Study the drawing (mm; zero at the part's minimum x, y, z) and answer. Give positions to 0.01 mm unless a question says otherwise; leave off trailing zeros. Order: outer loops, then holes, each group sorted by start corner. A loop starts at its lowest first (then second) coordinate and runs counter-clockwise, first axis right, second up.
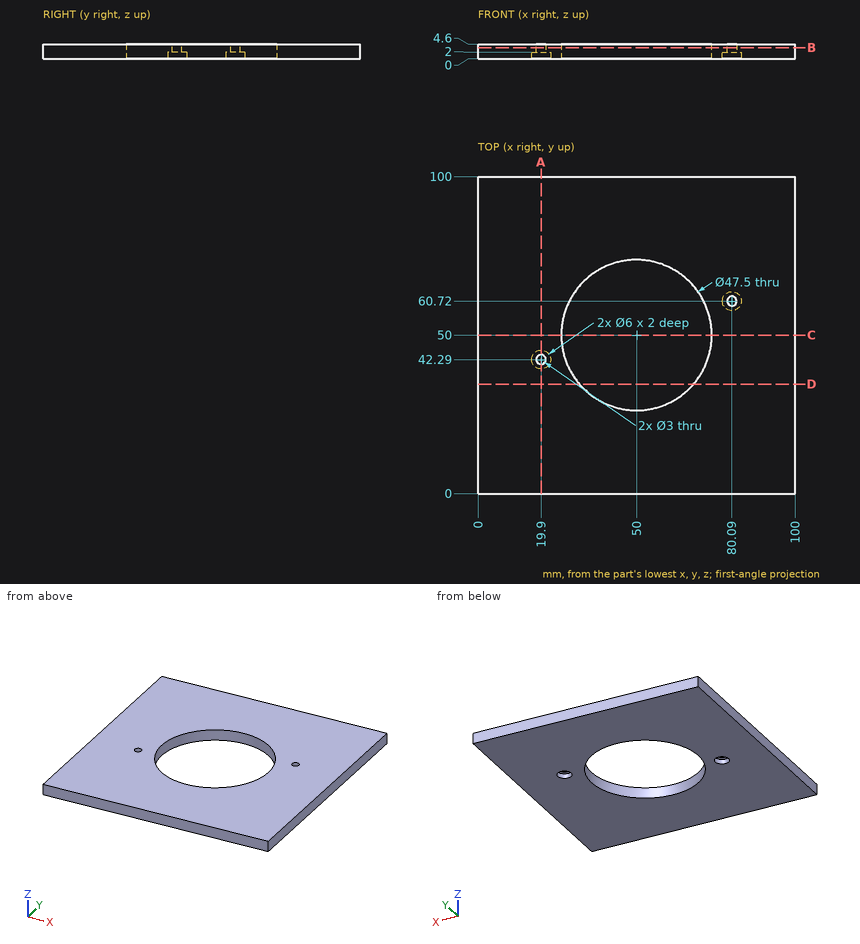
1) Given P1, Ø3.5, axis at x = 80.09, y = 60.72, coming from the -Z side, flat-ended and moving along its own axis, determine where the tip first touches the part or whether it passes through.
Geometry says:
P1: stops at z = 2
2) Find section C-C (y = 50). Write down the section's boundary in (x, z).
Geometry says:
outline: (0, 0) - (26.25, 0) - (26.25, 4.6) - (0, 4.6) - close; (73.75, 0) - (100, 0) - (100, 4.6) - (73.75, 4.6) - close
3) Find section B-B (z = 3.45). Write down the section's boundary in (x, y).
Geometry says:
outline: (0, 0) - (100, 0) - (100, 100) - (0, 100) - close; hole circle Ø3 at (19.9, 42.29); hole circle Ø47.5 at (50, 50); hole circle Ø3 at (80.09, 60.72)
4) Find section D-D (y = 34.5). Write down the section's boundary in (x, z), then the cut area to 3 significant figures.
Geometry says:
outline: (0, 0) - (32.01, 0) - (32.01, 4.6) - (0, 4.6) - close; (67.99, 0) - (100, 0) - (100, 4.6) - (67.99, 4.6) - close
area: 294 mm2
5) Find section A-A (x = 19.9). Write down the section's boundary in (y, z), then the cut area to 3 significant figures.
Geometry says:
outline: (0, 0) - (39.29, 0) - (39.29, 2) - (40.79, 2) - (40.79, 4.6) - (0, 4.6) - close; (43.79, 2) - (45.29, 2) - (45.29, 0) - (100, 0) - (100, 4.6) - (43.79, 4.6) - close
area: 440 mm2
6) Straight lines are drawn through the part: probe 1 along Y at (x, z) = (80.09, 3.55); probe 2 along Y at (x, z) = (19.9, 0.6); probe 3 along X at (y, z) = (49.5, 3.7). For each, find the intervals that lie inside material, in ascending order.
Geometry says:
probe 1: y = 0 to 59.22, 62.22 to 100
probe 2: y = 0 to 39.29, 45.29 to 100
probe 3: x = 0 to 26.26, 73.74 to 100
